Build history of the part. All positions in model axes, mm. Face numbers are marked on the shaded views. A direction names the side the tool comes from. Round coordinates to 2 decimals unless told otherwise and drop trailing zeros. Write each loop counter-clockwise with the first axis right and the second up, starting at its lowest first coordinate (ties: lowest second). Pieces come first, ordered by that corner, then holes. Notation, with made-up numbers: (78.25, 9.5) -> (132.25, 9.5) arc R17 cw to (132.25, 35.5) -> close; hole circle Ø1 at (-32, -27.5). An arc over 180 degrees is marked (long way). Answer in a Markdown table with one row per item.
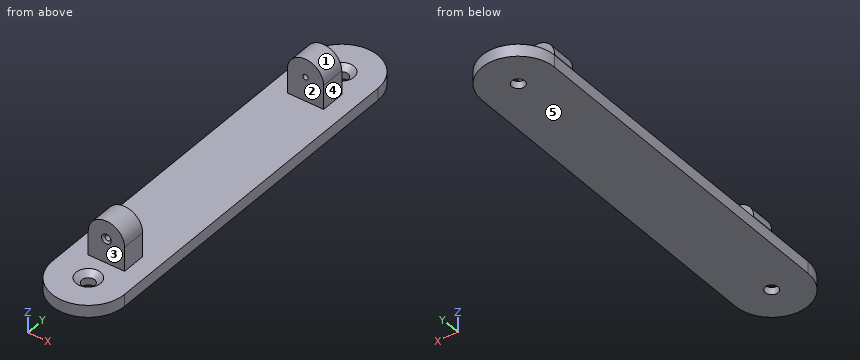
```python
from build123d import *

# Parameters (mm, degrees)
BOSS_EXTRUDE1_DEPTH                                 = 6.35
CSK_FOR_1_4_FLAT_HEAD_MACHINE_SCREW_100_D           = 6.7564
CSK_FOR_1_4_FLAT_HEAD_MACHINE_SCREW_100_CSINK_D     = 12.8778
CSK_FOR_1_4_FLAT_HEAD_MACHINE_SCREW_100_CSINK_ANGLE = 100
SKETCH8_W                                           = 19.05
SKETCH8_H                                           = 12.7
BOSS_EXTRUDE2_DEPTH                                 = 12.7
BOSS_EXTRUDE4_DEPTH                                 = 12.7
CSK_FOR_3_FLAT_HEAD_MACHINE_SCREW_100_D             = 2.794
CSK_FOR_3_FLAT_HEAD_MACHINE_SCREW_100_CSINK_D       = 5.0546
CSK_FOR_3_FLAT_HEAD_MACHINE_SCREW_100_CSINK_ANGLE   = 100


with BuildPart() as part:
    # Sketch2 → Boss-Extrude1 (new body)
    with BuildSketch(Plane.XY):
        with BuildLine():
            Line((0, 0), (0, 88.9))
            ThreePointArc((0, 88.9), (19.05, 107.95), (38.1, 88.9))
            Line((38.1, 88.9), (38.1, 0))
            Line((38.1, 0), (0, 0))
        make_face()
    extrude(amount=BOSS_EXTRUDE1_DEPTH)

    # CSK for 1/4 Flat Head Machine Screw (100)2 (through all)
    with Locations(Plane.XY.offset(6.35)):
        with Locations((19.05, 88.9)):
            CounterSinkHole(CSK_FOR_1_4_FLAT_HEAD_MACHINE_SCREW_100_D / 2, CSK_FOR_1_4_FLAT_HEAD_MACHINE_SCREW_100_CSINK_D / 2, counter_sink_angle=CSK_FOR_1_4_FLAT_HEAD_MACHINE_SCREW_100_CSINK_ANGLE)

    # Sketch8 → Boss-Extrude2 (add)
    with BuildSketch(Plane.XY.offset(6.35)):
        with Locations((19.05, 69.857100744)):
            Rectangle(SKETCH8_W, SKETCH8_H)
    extrude(amount=BOSS_EXTRUDE2_DEPTH)

    # Sketch10 → Boss-Extrude4 (add)
    with BuildSketch(Plane(origin=(0, 76.207100744, 0), x_dir=(1, 0, 0), z_dir=(0, 1, 0))):
        with BuildLine():
            Line((9.525, -19.05), (28.575, -19.05))
            ThreePointArc((28.575, -19.05), (19.05, -28.575), (9.525, -19.05))
        make_face()
    extrude(amount=-BOSS_EXTRUDE4_DEPTH)

    # CSK for #3 Flat Head Machine Screw (100)1 (through all)
    with Locations(Plane(origin=(0, 76.207100744, 0), x_dir=(1, 0, 0), z_dir=(0, 1, 0))):
        with Locations((19.05, -19.05)):
            CounterSinkHole(CSK_FOR_3_FLAT_HEAD_MACHINE_SCREW_100_D / 2, CSK_FOR_3_FLAT_HEAD_MACHINE_SCREW_100_CSINK_D / 2, counter_sink_angle=CSK_FOR_3_FLAT_HEAD_MACHINE_SCREW_100_CSINK_ANGLE)

    # Mirror1: part across plane


with BuildPart() as part_1:
    add(part.part)
    add(part.part.mirror(Plane(origin=(38.1, 0, 6.35), x_dir=(0, 0, 1), z_dir=(0, 1, 0))))


solid = part_1.part
```
Q1. Which spindle directions (+Z, -Z, +X, -X, +Y, -Y) get a long thin tool onto all of the face, cutting with end or side? Do the marked faces 1, 2, 3, 4 and 5. Say none if no direction does.
A:
| item | result |
|---|---|
| face 1 | +Z, +Y, -Y |
| face 2 | +Z, +X, -X |
| face 3 | +Z, +X, -X, -Y |
| face 4 | +Z, +X, +Y, -Y |
| face 5 | -Z, +X, -X, +Y, -Y |
Q2. Drop flat-ended pins along their axis: P1, Ø2.5, axis at x = 19.05, z = 19.05, coming from the -Y side; P2, Ø3.5, axis at x = 19.05, z = 19.05, coming from the +Y side; P3, Ø10, axis at y = 71, z = 15.5, coming from the -X side (3 decimals); P4, Ø12, axis at x = 16.5, y = 21.5, coming from the +Z side. Give the stop position or say it passes through.
A:
| item | result |
|---|---|
| P1 | through |
| P2 | y = 75.55 |
| P3 | x = 9.525 |
| P4 | z = 6.35 |
Q3. Saw through at D-D on y = -79. Write the cut outline in (x, z).
A:
| item | result |
|---|---|
| outline | (0, 0) -> (38.1, 0) -> (38.1, 6.35) -> (0, 6.35) -> close |
Q4. Saw through at B-B on z = 11.75. Write the cut outline in (x, y) (3 decimals), plus the area to 3 significant figures.
A:
| item | result |
|---|---|
| outline | (9.525, -76.207) -> (28.575, -76.207) -> (28.575, -63.507) -> (9.525, -63.507) -> close; (9.525, 63.507) -> (28.575, 63.507) -> (28.575, 76.207) -> (9.525, 76.207) -> close |
| area | 484 mm² |
Q5. Saw through at A-A on y = 66. Write the cut outline in (x, z) (3 decimals).
A:
| item | result |
|---|---|
| outline | (0, 0) -> (38.1, 0) -> (38.1, 6.35) -> (28.575, 6.35) -> (28.575, 19.05) arc R9.525 ccw to (9.525, 19.05) -> (9.525, 6.35) -> (0, 6.35) -> close; hole circle Ø2.794 at (19.05, 19.05) |
Q6. Wall check: line 1 (Y direction, x = 19.05, z = 1.2); line 2 (Z direction, x = 19.05, y = -73) (3 decimals); line 3 (Y direction, x = 27.5, z = 20.5). Give the ranges that are in metal, low to high. Write a range as [from, to].
A:
| item | result |
|---|---|
| line 1 | [-107.95, -92.28], [-85.52, 85.52], [92.28, 107.95] |
| line 2 | [0, 17.653], [20.447, 28.575] |
| line 3 | [-76.21, -63.51], [63.51, 76.21] |
Q7. Saw through at C-C on z = 25.5. Write the cut outline in (x, y), plus the area to 3 significant figures.
A:
| item | result |
|---|---|
| outline | (12.04, -76.21) -> (26.06, -76.21) -> (26.06, -63.51) -> (12.04, -63.51) -> close; (12.04, 63.51) -> (26.06, 63.51) -> (26.06, 76.21) -> (12.04, 76.21) -> close |
| area | 356 mm² |
